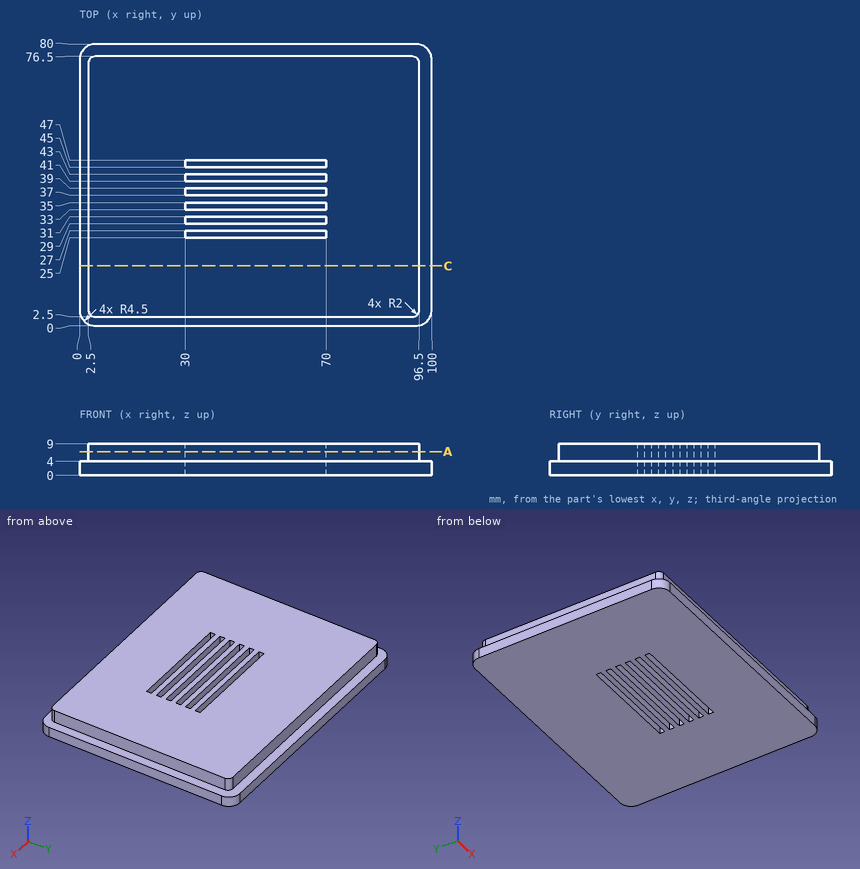
The figure shows three views and two pictorial views of one solid part (mm, origin at its lowest corner). Answer the questions. Round coordinates to 2 decimals unless told otherwise and drop trailing zeros. Order: outer loops, then holes, each group sorted by start corner. A loop starts at its lowest first (then second) coordinate and runs counter-clockwise, first axis right, second up.
Q1. A cutting plane is placed at A-A, the plane z = 6.75. Count the separate pieces of the cut face and the enclosed holes in it, then the cut area to 3 significant figures.
Solution:
separate pieces: 1
enclosed holes: 6
area: 6,470 mm2
Q2. Given pin 1 Ø2 at (x, y) = (48.5, 29) entering from -Z; pin 2 Ø4 at (y, z) = (55, 8) entering from -X; pin 3 Ø4 at (x, z) = (67.5, 6.5) entering from -Y; pin 4 Ø4 at (y, z) = (14, 7.5) entering from +X, each flat-ended and moving along its own axis, determine where each tip first touches the part or whether it passes through.
Solution:
pin 1: stops at z = 0
pin 2: stops at x = 2.5
pin 3: stops at y = 2.5
pin 4: stops at x = 96.5
Q3. Find the intervals of material crossed by line 1 along X through (y, z) = (45.5, 6.25); line 2 along Y through (x, z) = (16, 4.25); line 3 along X through (y, z) = (35.5, 4.5), in increasing order.
Solution:
line 1: x = 2.5 to 30, 70 to 96.5
line 2: y = 2.5 to 76.5
line 3: x = 2.5 to 96.5
Q4. A cutting plane is placed at C-C, the plane y = 17. Determine the outline of the cut face in (x, z).
Solution:
outline: (0, 0) - (100, 0) - (100, 4) - (96.5, 4) - (96.5, 9) - (2.5, 9) - (2.5, 4) - (0, 4) - close
